from build123d import *

# Parameters (mm, degrees)
SKETCH1_R           = 1.6
BOSS_EXTRUDE1_DEPTH = 3


with BuildPart() as part:
    # Sketch1 → Boss-Extrude1 (new body)
    with BuildSketch(Plane(origin=(0, 0, 0), x_dir=(1, 0, 0), z_dir=(0, 1, 0))):
        with BuildLine():
            ThreePointArc((-59.826654002, 10.230460246), (-63.30397667, 1.480635346), (-55.065238323, 6.038529506))
            add(Edge.make_bspline(
                [(-55.065238323, 6.038529506), (-46.710158882, 15.346176502), (-30, 24.653823498), (-13.289841118, 15.346176502), (-4.934761677, 6.038529506)],
                knots=[0.082246028, 0.082246028, 0.082246028, 0.082246028, 0.5, 0.917753972, 0.917753972, 0.917753972, 0.917753972], degree=3))
            ThreePointArc((-4.934761677, 6.038529506), (3.30397667, 1.480635346), (-0.173345998, 10.230460246))
            add(Edge.make_bspline(
                [(-59.826654002, 10.230460246), (-49.884436001, 23.410153415), (-30, 36.589846585), (-10.115563999, 23.410153415), (-0.173345998, 10.230460246)],
                knots=[0.0028891, 0.0028891, 0.0028891, 0.0028891, 0.5, 0.9971109, 0.9971109, 0.9971109, 0.9971109], degree=3))
        make_face()
        with Locations((-60, 5.233466033)):
            Circle(SKETCH1_R, mode=Mode.SUBTRACT)
        with Locations((0, 5.233466033)):
            Circle(SKETCH1_R, mode=Mode.SUBTRACT)
    extrude(amount=BOSS_EXTRUDE1_DEPTH)


solid = part.part
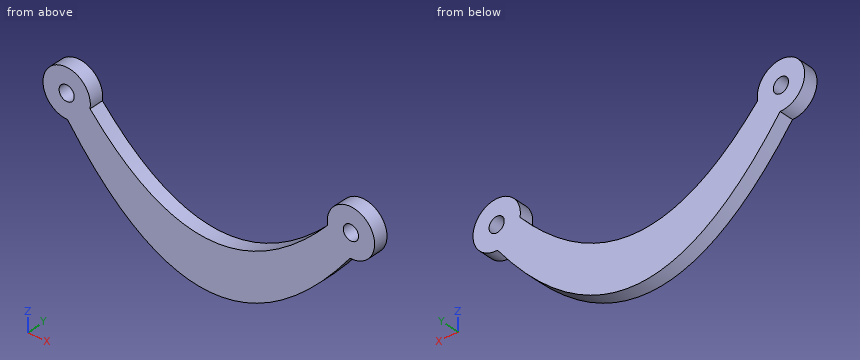
Geometry: final body of the model. Coordinates: model frame, mm. Give positions to 0.01 mm unless a question says otherwise; leave off trailing zeros. Answer in a Markdown table with one row per item. Add a question column.
(1) First-contact query: pin 1 (3 mm diameter, centred on x = -60, z = -5.23, fed in from -Y); pin 2 (4 mm diameter, centred on x = -39, z = -17.5, fed in from +Y). Flat tips, straight axial feed; report the tip coordinate or a pass-through.
(2) Section A-A on y = 1.1. State how many separate pieces and enclosed holes the cut face has, and give its area (3 significant figures).
(3) Ray query, line 1 (Z direction, x = -60, y = 1.1); line 2 (X direction, y = 1.1, z = -5); line 3 (X direction, y = 1.3, z = -8.5). Return the intervals inside material, ascending.
Result set:
| question | item | result |
|---|---|---|
| 1 | pin 1 | passes through |
| 1 | pin 2 | stops at y = 3 |
| 2 | separate pieces | 1 |
| 2 | enclosed holes | 2 |
| 2 | area | 681 mm^2 |
| 3 | line 1 | z = -10.23 to -6.83, -3.63 to -0.23 |
| 3 | line 2 | x = -64.99 to -61.58, -58.42 to -55.01, -4.99 to -1.58, 1.58 to 4.99 |
| 3 | line 3 | x = -63.79 to -52.75, -7.25 to 3.79 |
